The model under review builds one solid part; all positions refer to its coordinate system, in mm. A direction names the side the tool comes from. Give positions to 0.01 mm unless a question says otherwise; leave off trailing zeros. Write each loop counter-clockwise with the first axis right and the second up, starting at its lowest first coordinate (ties: lowest second). Pieces come first, ordered by that corner, then holes. Notation, with made-up numbers: (-24, 25) -> (-18, 25) arc R25 ccw to (-18, 43) -> close; hole circle Ø4 at (60, 66.5). An arc over 180 degrees is marked (long way). Use CSV: the item, a comma, the result in double quotes.
```python
from build123d import *

# Parameters (mm, degrees)
BASPROSKE_W         = 5.08
BASPROSKE_H         = 17.78
TOOTHCUT_DEPTH      = 26.652742543
TEETHCUTS_COUNT     = 26
TEETHCUTS_ANGLE     = 346.153846154
BORSKE_R            = 0.99949
BORE_DEPTH          = 50.8000508
SKETCH1_R           = 0.99949
BOSS_EXTRUDE1_DEPTH = 5.08
SKETCH2_R           = 4.269994
BOSS_EXTRUDE2_DEPTH = 13.97
SKETCH3_R           = 2.649982
CUT_EXTRUDE1_DEPTH  = 3.81


with BuildPart() as part:
    # BasProSke → Base-Revolve (revolve)
    with BuildSketch(Plane(origin=(0, 0, 0), x_dir=(1, 0, 0), z_dir=(0, 1, 0)), mode=Mode.PRIVATE) as base_revolve_sk:
        with Locations((2.54, 8.89)):
            Rectangle(BASPROSKE_W, BASPROSKE_H)
    revolve(base_revolve_sk.sketch.rotate(Axis((-10, 0, 0), (1, 0, 0)), 180), axis=Axis((-10, 0, 0), (1, 0, 0)))

    # TooCutSke → ToothCut (cut, through all)
    with BuildSketch(Plane(origin=(0, 0, 0), x_dir=(0, 0, -1), z_dir=(1, 0, 0))):
        with BuildLine():
            ThreePointArc((0.612177536, 14.922648482), (0, 14.9352), (-0.612177536, 14.922648482))
            ThreePointArc((-0.612177536, 14.922648482), (-1.047858816, 16.387671439), (-1.808659463, 17.713300655))
            ThreePointArc((-1.808659463, 17.713300655), (0, 17.8054), (1.808659463, 17.713300655))
            ThreePointArc((1.808659463, 17.713300655), (1.047858816, 16.387671439), (0.612177536, 14.922648482))
        make_face()
    toothcut = extrude(amount=TOOTHCUT_DEPTH, mode=Mode.SUBTRACT)

    # TeethCuts: ToothCut ×26 about axis
    teethcuts_axis = Axis((-10, 0, 0), (1, 0, 0))
    for i in range(1, TEETHCUTS_COUNT):
        add(toothcut.rotate(teethcuts_axis, i * TEETHCUTS_ANGLE / (TEETHCUTS_COUNT - 1)), mode=Mode.SUBTRACT)

    # BorSke → Bore (cut, symmetric)
    with BuildSketch(Plane(origin=(0, 0, 0), x_dir=(0, 0, -1), z_dir=(1, 0, 0))):
        with Locations(Location((0, 0, 0), (0, 0, 180))):
            Circle(BORSKE_R)
    extrude(amount=BORE_DEPTH, both=True, mode=Mode.SUBTRACT)

    # Sketch1 → Boss-Extrude1 (add)
    with BuildSketch(Plane(origin=(5.08, 0, 0), x_dir=(0, 0, -1), z_dir=(1, 0, 0))):
        Circle(SKETCH1_R)
    extrude(amount=-BOSS_EXTRUDE1_DEPTH)

    # Sketch2 → Boss-Extrude2 (add)
    with BuildSketch(Plane.ZY):
        with Locations(Location((0, 0, 0), (0, 0, 180))):
            Circle(SKETCH2_R)
    extrude(amount=BOSS_EXTRUDE2_DEPTH)

    # Sketch3 → Cut-Extrude1 (cut)
    with BuildSketch(Plane.ZY.offset(13.97)):
        Circle(SKETCH3_R)
    extrude(amount=-CUT_EXTRUDE1_DEPTH, mode=Mode.SUBTRACT)


solid = part.part
```
Q1. Machinability: for faces 1 (the cylindrical face through (2.504, -1.792, 14.827)), 2 (the cylindrical face through (2.504, -0.945, -16.36)), 3 (the cylindrical face through (2.5, 8.45, -14.09)), 4 (the cylindrical face through (2.5, -16.35, -1.03)), which of the approach directions +Z, -Z, +X, -X, +Y, -Y give a long, thin tool a straight path to every point of the face, cutting with its end or side? Answer none if there is none.
Derived:
face 1,"+Z, +X, -X"
face 2,"-Z, +X, -X"
face 3,"+X, -X"
face 4,"+X, -X, -Y"
Q2. Consider section B-B (x = -12.5). Write out the cut boundary in (y, z).
Derived:
outline,"circle Ø8.54 at (0, 0); hole circle Ø5.3 at (0, 0)"
Q3. The part is to be moulded in two halves that separate along Y. For faces 5 (the flat face through (-10.16, 0, 0)), 6 (the cylindrical face through (2.504, -14.001, -8.516)), 7 (the flat face through (5.08, 0, 0)), say which applies: pulls with the +Y half, pulls with the -Y half, needs draft (parallel to the pull), parting line crosses it, or undercut.
Derived:
face 5,"undercut"
face 6,"pulls with the -Y half"
face 7,"needs draft"
Q4. Consider section A-A (z = 0). Write out the cut boundary in (x, y), then the cut area to 3 significant figures.
Derived:
outline,"(-13.97, -4.27) -> (0, -4.27) -> (0, -14.94) -> (5.08, -14.94) -> (5.08, 14.94) -> (0, 14.94) -> (0, 4.27) -> (-13.97, 4.27) -> (-13.97, 2.65) -> (-10.16, 2.65) -> (-10.16, -2.65) -> (-13.97, -2.65) -> close"
area,"251 mm2"
Q5. To check wall thickness, follow probe 1 along Y at (x, z) = (-11.8, 0); probe 2 along Z at (x, y) = (0.75, -11.5); probe 3 along Y at (x, z) = (1.75, -13). State the ranges of each line that lie inside material, in increasing order.
Derived:
probe 1,"y = -4.27 to -2.65, 2.65 to 4.27"
probe 2,"z = -13.53 to -11.5, -9.53 to 9.53, 11.5 to 13.53"
probe 3,"y = -12.04 to -10.35, -8.13 to 8.13, 10.35 to 12.04"
Q6. Consider section C-C (x = -8.25). Write out the cut boundary in (y, z).
Derived:
outline,"circle Ø8.54 at (0, 0)"
Q7. Insertion check: pin 1 (1 mm diameter, centred on x = 2, z = -6, fed in from +Y); pin 2 (1 mm diameter, centred on x = -5.5, y = 1.5, fed in from -Z); pin 3 (1.5 mm diameter, centred on x = -1.5, z = -4, fed in from +Y). Each pin has a flat end and moves straight along its axis. Give the tip position at first contact, or say it passes through.
Derived:
pin 1,"stops at y = 16.75"
pin 2,"stops at z = -4.15"
pin 3,"stops at y = 2.77"
Q8. Consider section D-D (y = 6.5). Write out the cut boundary in (x, z), then the cut area to 3 significant figures.
Derived:
outline,"(0, -14.63) -> (5.08, -14.63) -> (5.08, 14.63) -> (0, 14.63) -> close"
area,"149 mm2"
